Check sheet for the modelled part. Datum: model origin and axes. Units: mm. A direction names the side the tool comes from. Round coordinates to 2 decimals unless told otherwise and drop trailing zeros. Write each loop counter-clockwise with the first axis right and the second up, starting at its lowest first coordinate (ties: lowest second). Pieces come first, ordered by that corner, then holes. Notation, with made-up numbers: (62, -12) - (88, -12) arc R14 ccw to (88, 5) - close; hole circle Ø8 at (5, -33). An arc over 180 degrees is marked (long way). Use one line per item in the form item = value. Start each with the question number.
1) Section check D-D (y = 2.65). Record the boundary of the cut face in (x, z).
2) Draft check along X on faces 1 (the face through (-2.5, 2, 0)), 2 (the face through (-1.5, 3, 0)), 3 (the face through (2, 5, 0)). Enter one of: +X half, -X half, draft (parallel to the pull), parting line (faces both ways), or undercut.
3) Section check C-C (x = 0). Record the boundary of the cut face in (y, z), then the cut area to 3 significant figures.
4) Gauge pin test, flat ends, axial feed: P1, Ø1.5, axis at y = 4, z = 1, coming from the +X side; P2, Ø0.5, axis at y = 3, z = 2, coming from the +X side; P3, Ø1.5, axis at y = 2, z = 0, coming from the -X side. Record the tip position at first contact, or that the pin passes through.
5) Set-up check for faces 4 (the face through (0, 0, 0)), 5 (the face through (0, 1, 0)), 6 (the face through (1, 4, 2)): record each of +Z, -Z, +X, -X, +Y, -Y from which the full face is reachable in a straight line by a thin tool's end or side.
6) Section check A-A (y = 4). Record the boundary of the cut face in (x, z).
7) Section check B-B (z = -1.15). Record the boundary of the cut face in (x, y).
8) Scan lines: probe 1 along X at (y, z) = (4.5, -1.05); probe 2 along X at (y, z) = (4, -0.2). Record each from-to range of solid material in increasing order.
Autodesk Inventor part; units mm, degrees
ref_plane "YZ Plane" through (0, 0, 0) normal (1, 0, 0) x (0, 1, 0)
ref_plane "XZ Plane" through (0, 0, 0) normal (0, 1, 0) x (-1, 0, 0)
ref_plane "XY Plane" through (0, 0, 0) normal (0, 0, 1) x (1, 0, 0)
sketch "Sketch1" plane through (0, 0, 0) normal (0, 1, 0) x (-1, 0, 0)
  line L0 (-2.5, 2.5) -> (2.5, 2.5)
  line L1 (2.5, 2.5) -> (2.5, -2.5)
  line L2 (2.5, -2.5) -> (-2.5, -2.5)
  line L3 (-2.5, -2.5) -> (-2.5, 2.5)
  line L4 (-2.5, 2.5) -> (2.5, -2.5) construction
  line L5 (2.5, 2.5) -> (-2.5, -2.5) construction
  point P0 (0, 0)
  dimension "d0" = 5
  dimension "d1" = 5
extrude "Extrusion1" add sketch "Sketch1" along normal blind 5
shell "Shell1" thickness 1 removed faces 1 at (-0.8333, 5, -0.8333)
sketch "Sketch3" plane through (-2.5, 0, 2.5) normal (0, 0, 1) x (1, 0, 0)
  line L0 (2.5, 9.1674) -> (2.5, 2.1156) construction
  line L1 (1.4995, 9.1674) -> (1.4995, 2.1156)
  line L2 (3.5005, 2.1156) -> (3.5005, 9.1674)
  arc A0 (3.5005, 9.1674) -> (1.4995, 9.1674) centre (2.5, 9.1674) ccw
  arc A1 (1.4995, 2.1156) -> (3.5005, 2.1156) centre (2.5, 2.1156) ccw
  point P0 (2.5, 0)
  point P1 (2.5, 5.6415)
extrude "Extrusion3" cut sketch "Sketch3" against normal through all
sketch "Sketch4" plane through (0, 5, 0) normal (0, 1, 0) x (1, 0, 0)
  point P0 (0, 0)
sketch "Sketch5" plane through (0, 5, 0) normal (0, 1, 0) x (1, 0, 0)
  point P0 (0, 0)
sketch "Sketch6" plane through (0, 5, 0) normal (0, 1, 0) x (1, 0, 0)
  point P0 (0, 0)
sketch "Sketch7" plane through (0, 0, 0) normal (0, -1, 0) x (1, 0, 0)
  point P0 (0, 0)
sketch "Sketch8" plane through (-2.5, 0, -2.5) normal (-1, 0, 0) x (0, 0, 1)
  point P0 (2.5, 0)
sketch "Sketch9" plane through (2.5, 0, 2.5) normal (1, 0, 0) x (0, 0, -1)
  line L0 (1.5, 3.5) -> (3.5, 3.5)
  line L1 (3.5, 3.5) -> (3.5, 4.5)
  line L2 (3.5, 4.5) -> (1.5, 4.5)
  line L3 (1.5, 4.5) -> (1.5, 3.5)
  line L4 (1.5, 3.5) -> (3.5, 4.5) construction
  line L5 (3.5, 3.5) -> (1.5, 4.5) construction
  line L6 (0, 5) -> (5, 5)
  point P0 (2.5, 0)
  point P1 (2.5, 4)
  dimension "d10" = 1
  dimension "d14" = 2
  dimension "d15" = 1
extrude "Extrusion4" add sketch "Sketch9" along normal blind 0.2 draft -60
sketch "Sketch10" plane through (-2.5, 0, -2.5) normal (-1, 0, 0) x (0, 0, 1)
  line L0 (1.5, 3.5) -> (3.5, 3.5)
  line L1 (3.5, 3.5) -> (3.5, 4.5)
  line L2 (3.5, 4.5) -> (1.5, 4.5)
  line L3 (1.5, 4.5) -> (1.5, 3.5)
  line L4 (1.5, 3.5) -> (3.5, 4.5) construction
  line L5 (3.5, 3.5) -> (1.5, 4.5) construction
  line L6 (0, 5) -> (5, 5)
  point P0 (2.5, 0)
  point P1 (2.5, 4)
  dimension "d13" = 1
  dimension "d16" = 2
  dimension "d17" = 1
extrude "Extrusion5" add sketch "Sketch10" along normal blind 0.2 draft -60
equation "\"d16\" = d14"
equation "\"d17\" = d15"
properties part number "snapfit_v08"
Results are:
q1.outline = (-2.5, -2.5) - (-1, -2.5) - (-1, -1.5) - (-1.5, -1.5) - (-1.5, 1.5) - (-1, 1.5) - (-1, 2.5) - (-2.5, 2.5) - close; (1, -2.5) - (2.5, -2.5) - (2.5, 2.5) - (1, 2.5) - (1, 1.5) - (1.5, 1.5) - (1.5, -1.5) - (1, -1.5) - close
q2.face_1 = -X half
q2.face_2 = undercut
q2.face_3 = draft
q3.outline = (0, -2.5) - (1.12, -2.5) - (1.12, -1.5) - (1, -1.5) - (1, 1.5) - (1.12, 1.5) - (1.12, 2.5) - (0, 2.5) - close
q3.area = 5.23 mm²
q4.P1 = 2.7
q4.P2 = 2.5
q4.P3 = -2.5
q5.face_4 = +Z, -Z, +X, -X, -Y
q5.face_5 = +Y
q5.face_6 = +Z, -Z, +Y
q6.outline = (-2.7, -0.65) - (-2.5, -1) - (-2.5, -2.5) - (-1, -2.5) - (-1, -1.5) - (-1.5, -1.5) - (-1.5, 1.5) - (-1, 1.5) - (-1, 2.5) - (-2.5, 2.5) - (-2.5, 1) - (-2.7, 0.65) - close; (1, -2.5) - (2.5, -2.5) - (2.5, -1) - (2.7, -0.65) - (2.7, 0.65) - (2.5, 1) - (2.5, 2.5) - (1, 2.5) - (1, 1.5) - (1.5, 1.5) - (1.5, -1.5) - (1, -1.5) - close
q7.outline = (-2.5, 0) - (2.5, 0) - (2.5, 5) - (1.5, 5) - (1.5, 1) - (-1.5, 1) - (-1.5, 5) - (-2.5, 5) - close
q8.probe_1 = -2.5 to -1.5, 1.5 to 2.5
q8.probe_2 = -2.7 to -1.5, 1.5 to 2.7
